Model file for the job. Use its own axes, mm. Coordinates: 2 decimals unless noted, no trailing zeros. Write each loop counter-clockwise with the first axis right and the second up, starting at its lowest first coordinate (ties: lowest second). Pieces come first, ordered by that corner, then holes. Notation, with made-up numbers: M -36.5,-18.5 L -2.5,-18.5 A9 ccw -2.5,-11.5 Z; hole C 51,48 d6. An arc over 180 degrees is marked long. Answer in a Markdown table with one row per item. Add a question column.
Autodesk Inventor part; units mm, degrees
ref_plane "YZ Plane" through (0, 0, 0) normal (1, 0, 0) x (0, 1, 0)
ref_plane "XZ Plane" through (0, 0, 0) normal (0, 1, 0) x (-1, 0, 0)
ref_plane "XY Plane" through (0, 0, 0) normal (0, 0, 1) x (1, 0, 0)
sketch "Sketch2" plane through (0, 0, 0) normal (0, 1, 0) x (-1, 0, 0)
  line L0 (12.7, 25.4) -> (-12.7, 25.4)
  line L1 (-12.7, 25.4) -> (-12.7, -25.4)
  line L2 (-12.7, -25.4) -> (12.7, -25.4)
  line L3 (12.7, -25.4) -> (12.7, 25.4)
  line L4 (12.7, 25.4) -> (-12.7, -25.4) construction
  line L5 (-12.7, 25.4) -> (12.7, -25.4) construction
  point P0 (0, 0)
  dimension "d0" = 25.4
  dimension "d1" = 50.8
extrude "Extrusion1" add sketch "Sketch2" along normal blind 19.05
sketch "Sketch3" plane through (0, 19.05, 0) normal (0, 1, 0) x (1, 0, 0)
  point P0 (0, 0)
  point P1 (0, -12.7)
  point P2 (0, 0)
  point P3 (0, 12.7)
  dimension "d4" = 12.7
  dimension "d5" = 12.7
hole "Hole1" at (0, 19.05, 12.7) at (0, 19.05, 0) at (0, 19.05, -12.7) direction (0, -1, 0) diameter 5.1054 end through all
properties part number "CL4-022" material "Aluminum 6061"
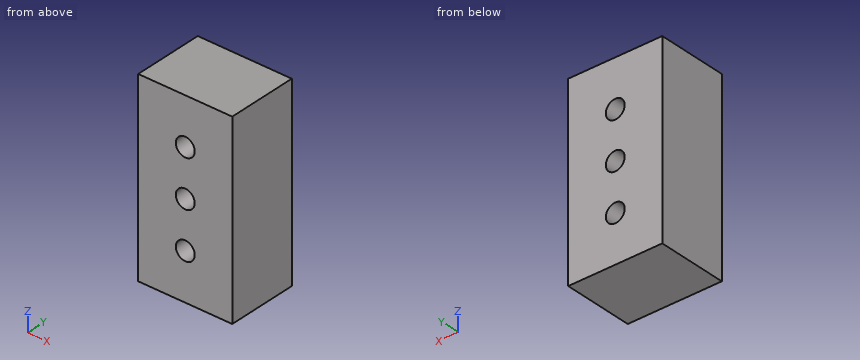
1) Drill centre lines: probe 1 along Z at (x, y) = (0, 13); probe 2 along Z at (x, y) = (-0.25, 15.5); probe 3 along X at (y, z) = (10, -12.7). Where is each one in solid material? Low to high.
2) Slice it at A-A (x = 0). Give the cut face in (y, z), then the cut area to 3 significant figures.
3) Slice it at C-C (z = 12.7). Give the cut face in (x, y), then the cut area to 3 significant figures.
4) Slice it at B-B (y = 10.5). Give the cut face in (x, z), then the cut area to 3 significant figures.
Ans:
| question | item | result |
|---|---|---|
| 1 | probe 1 | z = -25.4 to -15.25, -10.15 to -2.55, 2.55 to 10.15, 15.25 to 25.4 |
| 1 | probe 2 | z = -25.4 to -15.24, -10.16 to -2.54, 2.54 to 10.16, 15.24 to 25.4 |
| 1 | probe 3 | x = -12.7 to -2.55, 2.55 to 12.7 |
| 2 | outline | M 0,-25.4 L 19.05,-25.4 L 19.05,-15.25 L 0,-15.25 Z; M 0,-10.15 L 19.05,-10.15 L 19.05,-2.55 L 0,-2.55 Z; M 0,2.55 L 19.05,2.55 L 19.05,10.15 L 0,10.15 Z; M 0,15.25 L 19.05,15.25 L 19.05,25.4 L 0,25.4 Z |
| 2 | area | 676 mm2 |
| 3 | outline | M -12.7,0 L -2.55,0 L -2.55,19.05 L -12.7,19.05 Z; M 2.55,0 L 12.7,0 L 12.7,19.05 L 2.55,19.05 Z |
| 3 | area | 387 mm2 |
| 4 | outline | M -12.7,-25.4 L 12.7,-25.4 L 12.7,25.4 L -12.7,25.4 Z; hole C 0,-12.7 d5.11; hole C 0,0 d5.11; hole C 0,12.7 d5.11 |
| 4 | area | 1,230 mm2 |
